Source: three-view drawing plus pictorial views. Frame: mm from the lowest corner of the part. Give positions to 0.01 mm unless a question says otherwise; leave off trailing zeros. Loops run counter-clockwise (first coordinate to the right, second up) from the corner with the lowest first, then second, coordinate; pieces in that order, holes last. Notation, with made-up numbers: (38.5, 19.25) -> (91.5, 19.25) arc R12 cw to (91.5, 35.25) -> close; hole circle Ø11 at (-26, 11). An arc over 180 degrees is marked (long way). Put each result on its own line as item: value.
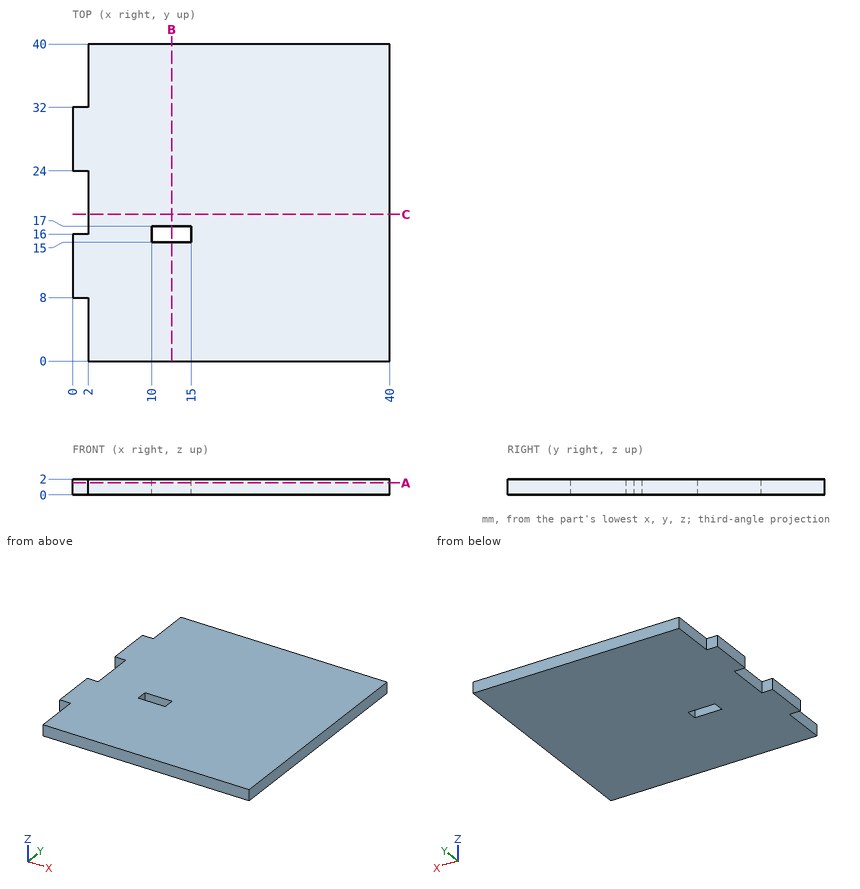
(1) First-contact query: P1, Ø1, axis at y = 21.5, z = 1.5, coming from the -X side; P2, Ø0.6, axis at x = 0.5, z = 1.5, coming from the +Y side; P3, Ø0.6, axis at x = 1.5, z = 1, coming from the -Y side. Flat tips, straight axial feed; report the tip coordinate or a pass-through.
Calculated:
P1: stops at x = 2
P2: stops at y = 32
P3: stops at y = 8
(2) Line query: probe 1 along Y at (x, z) = (12.5, 0.75); probe 2 along X at (y, z) = (18, 1.5). Output: solid intervals per line, ascending. Write a range as from..to.
Calculated:
probe 1: y = 0..15, 17..40
probe 2: x = 2..40
(3) Section A-A on z = 1.5. Return loops of the section in (x, y), then the cut area to 3 significant figures.
Calculated:
outline: (0, 8) -> (2, 8) -> (2, 0) -> (40, 0) -> (40, 40) -> (2, 40) -> (2, 32) -> (0, 32) -> (0, 24) -> (2, 24) -> (2, 16) -> (0, 16) -> close; hole (10, 15) -> (15, 15) -> (15, 17) -> (10, 17) -> close
area: 1,540 mm²
(4) Section B-B on x = 12.5. Return loops of the section in (y, z), then the cut area to 3 significant figures.
Calculated:
outline: (0, 0) -> (15, 0) -> (15, 2) -> (0, 2) -> close; (17, 0) -> (40, 0) -> (40, 2) -> (17, 2) -> close
area: 76.0 mm²
(5) Section C-C on y = 18.5. Return loops of the section in (x, z).
Calculated:
outline: (2, 0) -> (40, 0) -> (40, 2) -> (2, 2) -> close
